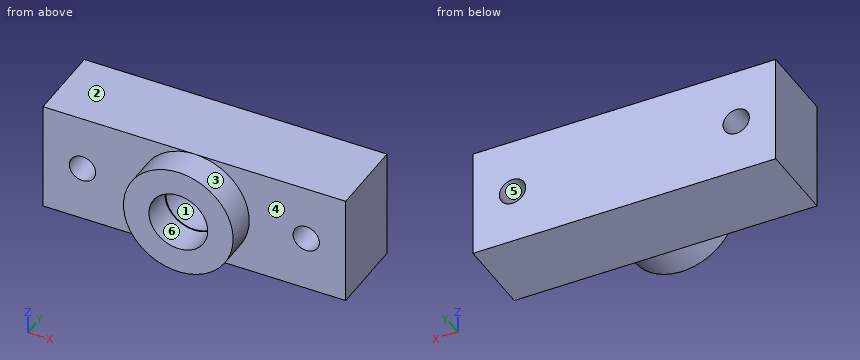
```python
from build123d import *

# Parameters (mm, degrees)
F0_W     = 34.5
F0_H     = 12.5
F0_R     = 1.5
F0_R_2   = 3.25
F1_DEPTH = 9
F2_R     = 6.25
F2_R_2   = 3.35
F3_DEPTH = 3.5
F4_W     = 10.950644
F4_H     = 8.111588
F5_DEPTH = 2


with BuildPart() as f1:
    # F0 (on Front) → F1 (new body)
    with BuildSketch(Plane.XZ):
        Rectangle(F0_W, F0_H)
        with Locations((-12.75, 0)):
            Circle(F0_R, mode=Mode.SUBTRACT)
        Circle(F0_R_2, mode=Mode.SUBTRACT)
        with Locations((12.75, 0)):
            Circle(F0_R, mode=Mode.SUBTRACT)
    extrude(amount=F1_DEPTH)

    # F2 (on face) → F3 (join)
    with BuildSketch(Plane.XZ.offset(9)):
        Circle(F2_R)
        Circle(F2_R_2, mode=Mode.SUBTRACT)
    extrude(amount=F3_DEPTH)

    # F4 (on face) → F5 (join)
    with BuildSketch(Plane(origin=(0, 0, 0), x_dir=(-1, 0, 0), z_dir=(0, 1, 0))):
        Rectangle(F4_W, F4_H)
    extrude(amount=-F5_DEPTH)


solid = f1.part
```
Check sheet for the modelled part. Datum: model origin and axes. Units: mm. Face numbers are marked on the shaded views. A direction names the side the tool comes from. Give positions to 0.01 mm unless a question says otherwise; leave off trailing zeros. Write each loop counter-clockwise with the first axis right and the second up, starting at its lowest first coordinate (ties: lowest second). Pieces come first, ordered by that corner, then holes.
Item 1: Gauge pin test, flat ends, axial feed: pin 1 (2.5 mm diameter, centred on x = 12.75, z = 0, fed in from +Y); pin 2 (4 mm diameter, centred on x = 11.5, z = 0.5, fed in from -Y); pin 3 (1 mm diameter, centred on y = -10, z = -3, fed in from +X). Record the tip position at first contact, or that the pin passes through.
Item 2: Cross-section at B-B (x = 12.75). Enter the section's corners in (y, z).
Item 3: Draft check along Z on the marked faces 1, 2, 3 and 4. Enter one of: released by +Z, released by -Z, zero draft, split by the parting line, or undercut.
Item 4: Cross-section at D-D (z = -5). Enter the section's corners in (x, y).
Item 5: Scan lines: L1, parallel to Z at x = -12.75, y = -5.5; L2, parallel to Z at x = 0, y = -5; L3, parallel to X at y = -8, z = -1.25. Record each from-to range of solid material in increasing order.
Item 6: Cross-section at A-A (z = 0). Enter the section's corners in (x, y), and give its area (3 significant figures).
Item 7: Cross-section at C-C (y = -4.5). Enter the section's corners in (x, z), and give its area (3 significant figures).
Item 8: Access from +Z, -Z, +X, -X, +Y, -Y to the whole of each face (thin tool, end or side, straight path). Record for the marked faces 5 and 6.
Report:
1. pin 1: passes through
1. pin 2: stops at y = -9
1. pin 3: stops at x = 5.73
2. outline: (-9, -6.25) - (0, -6.25) - (0, -1.5) - (-9, -1.5) - close; (-9, 1.5) - (0, 1.5) - (0, 6.25) - (-9, 6.25) - close
3. face 1: undercut
3. face 2: released by +Z
3. face 3: split by the parting line
3. face 4: zero draft
4. outline: (-17.25, -9) - (-3.75, -9) - (-3.75, -12.5) - (3.75, -12.5) - (3.75, -9) - (17.25, -9) - (17.25, 0) - (-17.25, 0) - close
5. L1: z = -6.25 to -1.5, 1.5 to 6.25
5. L2: z = -6.25 to -3.25, 3.25 to 6.25
5. L3: x = -17.25 to -13.58, -11.92 to -3, 3 to 11.92, 13.58 to 17.25
6. outline: (-17.25, -9) - (-14.25, -9) - (-14.25, 0) - (-17.25, 0) - close; (-11.25, -9) - (-6.25, -9) - (-6.25, -12.5) - (-3.35, -12.5) - (-3.35, -9) - (-3.25, -9) - (-3.25, -2) - (3.25, -2) - (3.25, -9) - (3.35, -9) - (3.35, -12.5) - (6.25, -12.5) - (6.25, -9) - (11.25, -9) - (11.25, 0) - (-11.25, 0) - close; (14.25, -9) - (17.25, -9) - (17.25, 0) - (14.25, 0) - close
6. area: 231 mm2
7. outline: (-17.25, -6.25) - (17.25, -6.25) - (17.25, 6.25) - (-17.25, 6.25) - close; hole circle Ø3 at (-12.75, 0); hole circle Ø6.5 at (0, 0); hole circle Ø3 at (12.75, 0)
7. area: 384 mm2
8. face 5: +Y, -Y
8. face 6: -Y
